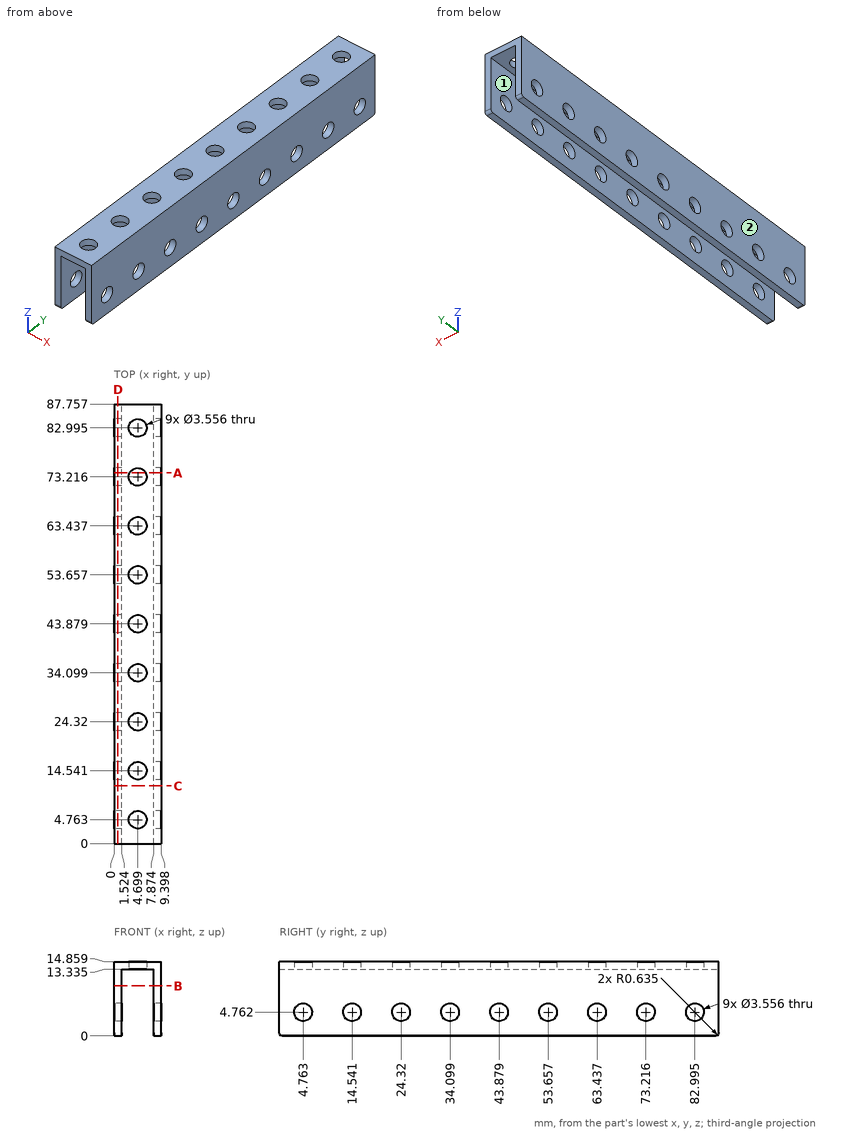
Can you work these out from the drawing? Everything is in mm from the part's minimum corner. A direction names the side the tool comes from. Round coordinates to 2 decimals unless told otherwise and drop trailing zeros. Loops run counter-clockwise (first coordinate to the right, second up) from the corner with the lowest first, then second, coordinate; pieces in that order, holes last. Notation, with made-up numbers: (42, 56) - (64, 56) arc R14 ccw to (64, 75) - close; hole circle Ø8 at (47, 22). An arc over 180 degrees is marked (long way). Answer in a Markdown table with one row per item. Add a question column.
(1) If we section it at D-D (x = 0.75): State how many separate pieces and enclosed holes the cut face has, plus the area to 3 significant figures.
(2) I need wall thicknesses on line 1 along X through (y, z) = (64.5, 1) (1 decimal); line 2 along Z through (x, y) = (4.25, 67) (1 decimal). Which ranges of each line are inside material? Lowest first, please.
(3) For the marked faces 1 and 2, which set-ups out of +Z, -Z, +X, -X, +Y, -Y let a thin tool reach every point of the face, with its end or its side?
(4) If we section it at B-B (z = 10): Please give me the cut outline in (x, y) (1 decimal).
(5) If we section it at A-A (y = 74): Please give me the cut outline in (x, z) (1 decimal).
(6) If we section it at C-C (y = 11.5): Please give me the cut outline in (x, z) (1 decimal).
(7) I'm going to push a flat-ended pin straight in: pin 1 (3 mm diameter, centred on x = 4.7, y = 43.88, fed in from -Z). Where does the tip first touch, or does it pass through?
Model answer:
| question | item | result |
|---|---|---|
| 1 | separate pieces | 1 |
| 1 | enclosed holes | 9 |
| 1 | area | 1,210 mm² |
| 2 | line 1 | x = 0 to 1.5, 7.9 to 9.4 |
| 2 | line 2 | z = 13.3 to 14.9 |
| 3 | face 1 | -Z, +Y, -Y |
| 3 | face 2 | +Z, -Z, -X, +Y, -Y |
| 4 | outline | (0, 0) - (1.5, 0) - (1.5, 87.8) - (0, 87.8) - close; (7.9, 0) - (9.4, 0) - (9.4, 87.8) - (7.9, 87.8) - close |
| 5 | outline | (0, 0) - (1.5, 0) - (1.5, 3.2) - (0, 3.2) - close; (0, 6.4) - (1.5, 6.4) - (1.5, 13.3) - (3.1, 13.3) - (3.1, 14.9) - (0, 14.9) - close; (6.3, 13.3) - (7.9, 13.3) - (7.9, 6.4) - (9.4, 6.4) - (9.4, 14.9) - (6.3, 14.9) - close; (7.9, 0) - (9.4, 0) - (9.4, 3.2) - (7.9, 3.2) - close |
| 6 | outline | (0, 0) - (1.5, 0) - (1.5, 13.3) - (7.9, 13.3) - (7.9, 0) - (9.4, 0) - (9.4, 14.9) - (0, 14.9) - close |
| 7 | pin 1 | passes through |
